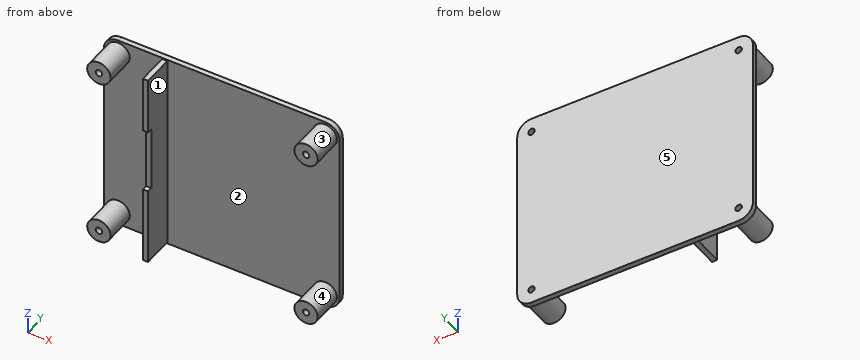
```python
from build123d import *

# Parameters (mm, degrees)
F1_DEPTH = 2
F2_R     = 4.5
F2_W     = 2
F2_H     = 77
F3_DEPTH = 12
F4_R     = 1.25
F5_DEPTH = 25
F6_W     = 2
F6_H     = 25
F7_DEPTH = 2


with BuildPart() as f1:
    # F0 (on Front) → F1 (new body)
    with BuildSketch(Plane.XZ):
        with BuildLine():
            Line((63, 77.5), (-17, 77.5))
            ThreePointArc((-17, 77.5), (-20.889087, 75.889087), (-22.5, 72))
            Line((-22.5, 72), (-22.5, 5))
            ThreePointArc((-22.5, 5), (-20.889087, 1.110913), (-17, -0.5))
            Line((-17, -0.5), (63, -0.5))
            ThreePointArc((63, -0.5), (66.889087, 1.110913), (68.5, 5))
            Line((68.5, 5), (68.5, 72))
            ThreePointArc((68.5, 72), (66.889087, 75.889087), (63, 77.5))
        make_face()
    extrude(amount=-F1_DEPTH)

    # F2 (on Front) → F3 (join)
    with BuildSketch(Plane.XZ):
        with Locations((-17, 72)):
            Circle(F2_R)
        with Locations((63, 72)):
            Circle(F2_R)
        with Locations((-17, 5)):
            Circle(F2_R)
        with Locations((63, 5)):
            Circle(F2_R)
        with Locations((1, 38.5)):
            Rectangle(F2_W, F2_H)
    extrude(amount=F3_DEPTH)

    # F4 (on face) → F5 (cut)
    with BuildSketch(Plane.XZ.offset(12)):
        with Locations((-17, 72)):
            Circle(F4_R)
        with Locations((63, 72)):
            Circle(F4_R)
        with Locations((63, 5)):
            Circle(F4_R)
        with Locations((-17, 5)):
            Circle(F4_R)
    extrude(amount=-F5_DEPTH, mode=Mode.SUBTRACT)

    # F6 (on face) → F7 (cut)
    with BuildSketch(Plane.XZ.offset(12)):
        with Locations((1, 42.5)):
            Rectangle(F6_W, F6_H)
    extrude(amount=-F7_DEPTH, mode=Mode.SUBTRACT)


solid = f1.part
```
The listing builds one solid part. Answer for the finished solid, in the listing's coordinates (mm). Face numbers are marked on the shaded views. A direction names the side the tool comes from. Round coordinates to 2 decimals unless told otherwise and drop trailing zeros. Order: outer loops, then holes, each group sorted by start corner. A loop starts at its lowest first (then second) coordinate and runs counter-clockwise, first axis right, second up. Notation, with made-up numbers: (67, 78.5) -> (74, 78.5) arc R14 cw to (74, 94.5) -> close; hole circle Ø9 at (-20, 34). An arc over 180 degrees is marked (long way). Answer as CSV lines item,"result". Start each with the question number.
(1) Find the intervals of material crossed by probe 1 along Z at (x, y) = (63, -8); probe 2 along X at (y, z) = (-1, 6.5); probe 3 along X at (y, z) = (-7.5, 6), in increasing order. Write a range as from..to.
(2) A tool of negligible diameter and unlimited length cuts with its end or side. For the marked faces 4 and 5, from which of +Z, -Z, +X, -X, +Y, -Y can it reach the whole face along a straight path? Write none if from no direction.
(3) The part is cut by section C-C (x = 28). Determine the outline of the cut face in (y, z), then the cut area to 3 significant figures.
(4) Flat-ended cylindrical pins translate along their axes: pin 1 Ø1 at (x, y) = (0.5, -8) entering from +Z; pin 2 Ø0.6 at (x, z) = (1, 40) entering from -Y; pin 3 Ø5 at (x, y) = (-4.5, -7) entering from -Z; pin 4 Ø2 at (x, y) = (1.5, -8) entering from -Z. Find the tip coordinate at first contact, or state that the pin passes through.
(5) The part is cut by section B-B (z = 60). Determine the outline of the cut face in (x, y), then the cut area to 3 significant figures.
(6) For a pull along Z with two mould halves and no side action, classify the marked faces 1, 2 and 3 as +Z half, -Z half, draft (parallel to the pull), parting line (faces both ways), or undercut.
(7) The part is cut by section A-A (y = -6.75). Count the separate pieces of the cut face and the enclosed holes in it, then the cut area to 3 significant figures.
Evaluation:
1,probe 1,"0.5..3.75, 6.25..9.5, 67.5..70.75, 73.25..76.5"
1,probe 2,"-21.24..-12.76, 0..2, 58.76..67.24"
1,probe 3,"-21.39..-17.75, -16.25..-12.61, 0..2, 58.61..62.25, 63.75..67.39"
2,face 4,"-Y"
2,face 5,"+Z, -Z, +X, -X, +Y"
3,outline,"(0, -0.5) -> (2, -0.5) -> (2, 77.5) -> (0, 77.5) -> close"
3,area,"156 mm²"
4,pin 1,"z = 77"
4,pin 2,"y = -10"
4,pin 3,"through"
4,pin 4,"z = 0"
5,outline,"(-22.5, 0) -> (0, 0) -> (0, -12) -> (2, -12) -> (2, 0) -> (68.5, 0) -> (68.5, 2) -> (-22.5, 2) -> close"
5,area,"206 mm²"
6,face 1,"draft"
6,face 2,"undercut"
6,face 3,"undercut"
7,separate pieces,"5"
7,enclosed holes,"4"
7,area,"389 mm²"
